from build123d import *

# Parameters (mm, degrees)
F1_DEPTH = 20.4
F4_DEPTH = 20
F5_DEPTH = 20
F7_DEPTH = 13
F8_DEPTH = 20.4
F9_DEPTH = 20.4


with BuildPart() as f1:
    # F0 (on Top) → F1 (new body)
    with BuildSketch(Plane.XY):
        Polygon((0, 40.4), (0, 0), (40.4, 0), (40.4, 20.4), (20.4, 20.4), (20.4, 40.4), align=None)
    extrude(amount=F1_DEPTH)

    # F3 (on face) → F4 (cut)
    with BuildSketch(Plane(origin=(0, 40.4, 0), x_dir=(-1, 0, 0), z_dir=(0, 1, 0))):
        with BuildLine():
            Line((-10.2, 10.2), (-2, 10.2))
            ThreePointArc((-2, 10.2), (-15.9982756057, 15.9982756057), (-10.2, 2))
            Line((-10.2, 2), (-10.2, 10.2))
        make_face()
        with BuildLine():
            ThreePointArc((-10.2, 2), (-4.4017243943, 4.4017243943), (-2, 10.2))
            Line((-2, 10.2), (-10.2, 10.2))
            Line((-10.2, 10.2), (-10.2, 2))
        make_face()
    extrude(amount=-F4_DEPTH, mode=Mode.SUBTRACT)

    # F2 (on face) → F5 (cut)
    with BuildSketch(Plane.YZ.offset(40.4)):
        with BuildLine():
            ThreePointArc((10.2, 2), (15.9982756057, 4.4017243943), (18.4, 10.2))
            Line((18.4, 10.2), (10.2, 10.2))
            Line((10.2, 10.2), (10.2, 2))
        make_face()
        with BuildLine():
            Line((10.2, 10.2), (18.4, 10.2))
            ThreePointArc((18.4, 10.2), (4.4017243943, 15.9982756057), (10.2, 2))
            Line((10.2, 2), (10.2, 10.2))
        make_face()
    extrude(amount=-F5_DEPTH, mode=Mode.SUBTRACT)

    # F6 (on face) → F7 (join)
    with BuildSketch(Plane.XY.offset(20.4)):
        with BuildLine():
            Line((18.2597766718, 0), (2.1402233282, 0))
            ThreePointArc((2.1402233282, 0), (10.2, -2.8), (18.2597766718, 0))
        make_face()
        with BuildLine():
            ThreePointArc((0, 18.2597766718), (-2.8, 10.2), (0, 2.1402233282))
            Line((0, 2.1402233282), (0, 18.2597766718))
        make_face()
        with BuildLine():
            Line((3.1289321881, 3.1289321881), (1.0076118446, 1.0076118446))
            ThreePointArc((1.0076118446, 1.0076118446), (1.5592177314, 0.4872824716), (2.1402233282, 0))
            Line((2.1402233282, 0), (18.2597766718, 0))
            ThreePointArc((18.2597766718, 0), (21.8999379642, 4.5333032874), (23.2, 10.2))
            ThreePointArc((23.2, 10.2), (22.2104339226, 15.1748846207), (19.3923881554, 19.3923881554))
            Line((19.3923881554, 19.3923881554), (17.2710678119, 17.2710678119))
            ThreePointArc((17.2710678119, 17.2710678119), (19.4387953251, 14.0268343237), (20.2, 10.2))
            ThreePointArc((20.2, 10.2), (14.0268343237, 0.9612046749), (3.1289321881, 3.1289321881))
        make_face()
        with BuildLine():
            ThreePointArc((0, 2.1402233282), (0.4872824716, 1.5592177314), (1.0076118446, 1.0076118446))
            Line((1.0076118446, 1.0076118446), (3.1289321881, 3.1289321881))
            ThreePointArc((3.1289321881, 3.1289321881), (3.1289321881, 17.2710678119), (17.2710678119, 17.2710678119))
            Line((17.2710678119, 17.2710678119), (19.3923881554, 19.3923881554))
            ThreePointArc((19.3923881554, 19.3923881554), (9.4420273089, 23.177884165), (0, 18.2597766718))
            Line((0, 18.2597766718), (0, 2.1402233282))
        make_face()
    extrude(amount=F7_DEPTH)

    # F6 (on face) → F8 (join)
    with BuildSketch(Plane.XY.offset(20.4)):
        with BuildLine():
            Line((18.2597766718, 0), (2.1402233282, 0))
            ThreePointArc((2.1402233282, 0), (10.2, -2.8), (18.2597766718, 0))
        make_face()
    extrude(amount=-F8_DEPTH)

    # F6 (on face) → F9 (join)
    with BuildSketch(Plane.XY.offset(20.4)):
        with BuildLine():
            ThreePointArc((0, 18.2597766718), (-2.8, 10.2), (0, 2.1402233282))
            Line((0, 2.1402233282), (0, 18.2597766718))
        make_face()
    extrude(amount=-F9_DEPTH)


solid = f1.part
Read the model definition and answer for the solid it produces. Units are mm, in the model's axes. A direction names the side the tool comes from. Give positions to 0.01 mm unless a question says otherwise; leave off trailing zeros. Loops run counter-clockwise (first coordinate to the right, second up) from the corner with the lowest first, then second, coordinate; pieces in that order, holes last. Notation, with made-up numbers: (-26.5, -17) - (7.5, -17) arc R23 ccw to (7.5, 20) - close; hole circle Ø11 at (34.25, 87.5). An arc over 180 degrees is marked (long way). Answer as CSV lines item,"result". Start each with the question number.
1) Find section D-D (y = 11). Write down the section's boundary in (x, z), then the cut area to 3 significant figures.
2) Which of the six approach directions +Z, -Z, +X, -X, +Y, -Y give full straight-line access (tool end or side, diameter ignored) to faces 1 (the face through (20.4, 30, 10)), 2 (the face through (10, 20.4, 10)), 3 (the face through (1, 0, 10)), 4 (the face through (0, 29, 10)), 5 (the face through (29, 0, 10))?
3) Determine the mould class of faces 6 (the face through (0, 1, 10)), 7 (the face through (20.4, 10, 10)), 8 (the face through (10, 10, 20.4)) for opening direction X: released by +X, released by -X, zero draft, split by the parting line, or undercut.
4) A straight line is drawn through the part: L1, parallel to Y at x = 26, z = 10.2. Find the intervals that lie inside material, in ascending order. Write a range as from..to.
5) Find section B-B (y = 36). Write down the section's boundary in (x, z), then the cut area to 3 significant figures.
6) Each of these flat-tipped pins is pushed along its axis until it touches: pin 1 Ø10 at (x, y) = (6.5, 7.5) entering from +Z; pin 2 Ø4 at (y, z) = (17.5, 14.5) entering from -X; pin 3 Ø3 at (y, z) = (19, 11.5) entering from -X. Where does it stop, or does it pass through?
7) Find section A-A (z = 24). Write down the section's boundary in (x, y).
Findings below:
1,outline,"(-2.78, 0) - (40.4, 0) - (40.4, 2.04) - (20.4, 2.04) - (20.4, 18.36) - (40.4, 18.36) - (40.4, 20.4) - (23.18, 20.4) - (23.18, 33.4) - (20.17, 33.4) - (20.17, 20.4) - (0.23, 20.4) - (0.23, 33.4) - (-2.78, 33.4) - close"
1,area,"633 mm^2"
2,face 1,"+Z, -Z, +X, +Y"
2,face 2,"+Y"
2,face 3,"+Z, -Z, -X, -Y"
2,face 4,"+Z, -Z, -X, +Y"
2,face 5,"+Z, -Z, +X, -Y"
3,face 6,"released by -X"
3,face 7,"released by +X"
3,face 8,"undercut"
4,L1,"0..2, 18.4..20.4"
5,outline,"(0, 0) - (20.4, 0) - (20.4, 20.4) - (0, 20.4) - close; hole circle Ø16.4 at (10.2, 10.2)"
5,area,"205 mm^2"
6,pin 1,"z = 20.4"
6,pin 2,"x = -1.67"
6,pin 3,"x = -0.56"
7,outline,"circle Ø26 at (10.2, 10.2); hole circle Ø20 at (10.2, 10.2)"
